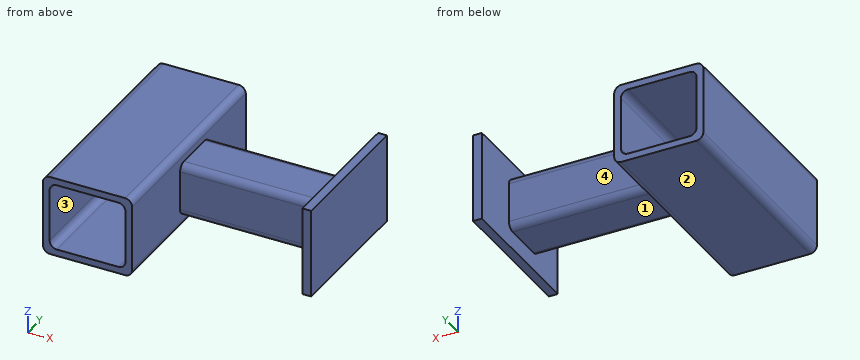
from build123d import *

# Parameters (mm, degrees)
F1_DEPTH = 152.4
F3_DEPTH = 101.6
F5_W     = 101.6
F5_H     = 63.5
F6_DEPTH = 6.35


with BuildPart() as f1:
    # F0 (on Front) → F1 (new body)
    with BuildSketch(Plane.XZ):
        with BuildLine():
            Line((-26.67, -28.575), (26.67, -28.575))
            ThreePointArc((26.67, -28.575), (30.2621024484, -27.0871024484), (31.75, -23.495))
            Line((31.75, -23.495), (31.75, 23.495))
            ThreePointArc((31.75, 23.495), (30.2621024484, 27.0871024484), (26.67, 28.575))
            Line((26.67, 28.575), (-26.67, 28.575))
            ThreePointArc((-26.67, 28.575), (-30.2621024484, 27.0871024484), (-31.75, 23.495))
            Line((-31.75, 23.495), (-31.75, -23.495))
            ThreePointArc((-31.75, -23.495), (-30.2621024484, -27.0871024484), (-26.67, -28.575))
        make_face()
        with BuildLine():
            Line((-21.9075, 23.8125), (21.9075, 23.8125))
            ThreePointArc((21.9075, 23.8125), (25.4996024484, 22.3246024484), (26.9875, 18.7325))
            Line((26.9875, 18.7325), (26.9875, -18.7325))
            ThreePointArc((26.9875, -18.7325), (25.4996024484, -22.3246024484), (21.9075, -23.8125))
            Line((21.9075, -23.8125), (-21.9075, -23.8125))
            ThreePointArc((-21.9075, -23.8125), (-25.4996024484, -22.3246024484), (-26.9875, -18.7325))
            Line((-26.9875, -18.7325), (-26.9875, 18.7325))
            ThreePointArc((-26.9875, 18.7325), (-25.4996024484, 22.3246024484), (-21.9075, 23.8125))
        make_face(mode=Mode.SUBTRACT)
    extrude(amount=-F1_DEPTH)

    # F2 (on face) → F3 (join)
    with BuildSketch(Plane.YZ.offset(31.75)):
        with BuildLine():
            Line((69.4262681528, -19.05), (97.3662681528, -19.05))
            ThreePointArc((97.3662681528, -19.05), (100.9583706013, -17.5621024484), (102.4462681528, -13.97))
            Line((102.4462681528, -13.97), (102.4462681528, 13.97))
            ThreePointArc((102.4462681528, 13.97), (100.9583706013, 17.5621024484), (97.3662681528, 19.05))
            Line((97.3662681528, 19.05), (69.4262681528, 19.05))
            ThreePointArc((69.4262681528, 19.05), (65.8341657044, 17.5621024484), (64.3462681528, 13.97))
            Line((64.3462681528, 13.97), (64.3462681528, -13.97))
            ThreePointArc((64.3462681528, -13.97), (65.8341657044, -17.5621024484), (69.4262681528, -19.05))
        make_face()
        with BuildLine():
            ThreePointArc((69.9342681528, -16.002), (68.1382169286, -15.2580512242), (67.3942681528, -13.462))
            Line((67.3942681528, -13.462), (67.3942681528, 13.462))
            ThreePointArc((67.3942681528, 13.462), (68.1382169286, 15.2580512242), (69.9342681528, 16.002))
            Line((69.9342681528, 16.002), (96.8582681528, 16.002))
            ThreePointArc((96.8582681528, 16.002), (98.6543193771, 15.2580512242), (99.3982681528, 13.462))
            Line((99.3982681528, 13.462), (99.3982681528, -13.462))
            ThreePointArc((99.3982681528, -13.462), (98.6543193771, -15.2580512242), (96.8582681528, -16.002))
            Line((96.8582681528, -16.002), (69.9342681528, -16.002))
        make_face(mode=Mode.SUBTRACT)
    extrude(amount=F3_DEPTH)

    # F4 (on face) + F5 (on face) → F6 (join)
    with BuildSketch(Plane.YZ.offset(133.35)):
        with BuildLine():
            ThreePointArc((64.3462681528, -13.97), (65.8341657044, -17.5621024484), (69.4262681528, -19.05))
            Line((69.4262681528, -19.05), (97.3662681528, -19.05))
            ThreePointArc((97.3662681528, -19.05), (100.9583706013, -17.5621024484), (102.4462681528, -13.97))
            Line((102.4462681528, -13.97), (102.4462681528, 13.97))
            ThreePointArc((102.4462681528, 13.97), (100.9583706013, 17.5621024484), (97.3662681528, 19.05))
            Line((97.3662681528, 19.05), (69.4262681528, 19.05))
            ThreePointArc((69.4262681528, 19.05), (65.8341657044, 17.5621024484), (64.3462681528, 13.97))
            Line((64.3462681528, 13.97), (64.3462681528, -13.97))
        make_face()
        with BuildLine():
            ThreePointArc((99.3982681528, -13.462), (98.6543193771, -15.2580512242), (96.8582681528, -16.002))
            Line((96.8582681528, -16.002), (69.9342681528, -16.002))
            ThreePointArc((69.9342681528, -16.002), (68.1382169286, -15.2580512242), (67.3942681528, -13.462))
            Line((67.3942681528, -13.462), (67.3942681528, 13.462))
            ThreePointArc((67.3942681528, 13.462), (68.1382169286, 15.2580512242), (69.9342681528, 16.002))
            Line((69.9342681528, 16.002), (96.8582681528, 16.002))
            ThreePointArc((96.8582681528, 16.002), (98.6543193771, 15.2580512242), (99.3982681528, 13.462))
            Line((99.3982681528, 13.462), (99.3982681528, -13.462))
        make_face(mode=Mode.SUBTRACT)
        with BuildLine():
            Line((69.9342681528, -16.002), (96.8582681528, -16.002))
            ThreePointArc((96.8582681528, -16.002), (98.6543193771, -15.2580512242), (99.3982681528, -13.462))
            Line((99.3982681528, -13.462), (99.3982681528, 13.462))
            ThreePointArc((99.3982681528, 13.462), (98.6543193771, 15.2580512242), (96.8582681528, 16.002))
            Line((96.8582681528, 16.002), (69.9342681528, 16.002))
            ThreePointArc((69.9342681528, 16.002), (68.1382169286, 15.2580512242), (67.3942681528, 13.462))
            Line((67.3942681528, 13.462), (67.3942681528, -13.462))
            ThreePointArc((67.3942681528, -13.462), (68.1382169286, -15.2580512242), (69.9342681528, -16.002))
        make_face()
    with BuildSketch(Plane.YZ.offset(133.35)):
        with Locations((87.8347480977, 0)):
            Rectangle(F5_W, F5_H)
        with BuildLine():
            ThreePointArc((102.4462681528, -13.97), (100.9583706013, -17.5621024484), (97.3662681528, -19.05))
            Line((97.3662681528, -19.05), (69.4262681528, -19.05))
            ThreePointArc((69.4262681528, -19.05), (65.8341657044, -17.5621024484), (64.3462681528, -13.97))
            Line((64.3462681528, -13.97), (64.3462681528, 13.97))
            ThreePointArc((64.3462681528, 13.97), (65.8341657044, 17.5621024484), (69.4262681528, 19.05))
            Line((69.4262681528, 19.05), (97.3662681528, 19.05))
            ThreePointArc((97.3662681528, 19.05), (100.9583706013, 17.5621024484), (102.4462681528, 13.97))
            Line((102.4462681528, 13.97), (102.4462681528, -13.97))
        make_face(mode=Mode.SUBTRACT)
    extrude(amount=F6_DEPTH)


solid = f1.part
CAD build for the part. Positions are in the model's coordinates, mm. Face numbers are marked on the shaded views. A direction names the side the tool comes from. Give positions to 0.01 mm unless a question says otherwise; leave off trailing zeros. Loops run counter-clockwise (first coordinate to the right, second up) from the corner with the lowest first, then second, coordinate; pieces in that order, holes last. Notation, with made-up numbers: M 54,23 L 65,23 A37 ccw 65,60 Z; hole C -24.5,85 d6. An arc over 180 degrees is marked long. One line per question, with ' | ' between items. Start each with the question number.
1. Saw through at B-B on x = -20. Give the cut face in (y, z) (1 decimal), plus the area to 3 significant figures.
2. Flat gauge pins, fed straight in: pin 1 (2 mm diameter, centred on x = 121, y = 85.5, fed in from +Z); pin 2 (5 mm diameter, centred on x = 28, z = -7, fed in from -Y); pin 3 (8 mm diameter, centred on x = 86.5, y = 86, fed in from -Z); pin 4 (13 mm diameter, centred on x = -9, y = 95.5, fed in from +Z) (3 decimals). Where does each tip first touch, or does it go through?
3. 3-axis set-ups, long thin cutter, end or side, ignore diameter. For the marked faces 1, 2, 3 and 4: which of +Z, -Z, +X, -X, +Y, -Y reach the whole face in a straight line?
4. Probe L1, parallel to X at y = 71, z = 9.5; L2, parallel to Z at x = 16.5, y = 49 (1 decimal); L3, parallel to Y at x = 88, z = 11. List the from-to ranges inside material, lowest first. Write a range as from..to.
5. Saw through at A-A on y = 41. State how many separate pieces and enclosed holes the cut face has, plus the area to 3 significant figures.
6. Saw through at C-C on x = 39.5. Give the cut face in (y, z), plus the area to 3 significant figures.
Result sheet:
1) outline: M 0,-28.6 L 152.4,-28.6 L 152.4,-23.8 L 0,-23.8 Z; M 0,23.8 L 152.4,23.8 L 152.4,28.6 L 0,28.6 Z | area: 1,450 mm^2
2) pin 1: stops at z = 19.05 | pin 2: stops at y = 0 | pin 3: stops at z = -19.05 | pin 4: stops at z = 28.575
3) face 1: -Z, +Y, -Y | face 2: -Z, -X, +Y, -Y | face 3: +Y, -Y | face 4: +Z, -Z, +Y
4) L1: x = -31.75..-26.99, 26.99..31.75, 133.35..139.7 | L2: z = -28.6..-23.8, 23.8..28.6 | L3: y = 64.35..67.39, 99.4..102.45
5) separate pieces: 2 | enclosed holes: 1 | area: 1,460 mm^2
6) outline: M 64.35,-13.97 A5.08 ccw 69.43,-19.05 L 97.37,-19.05 A5.08 ccw 102.45,-13.97 L 102.45,13.97 A5.08 ccw 97.37,19.05 L 69.43,19.05 A5.08 ccw 64.35,13.97 Z; hole M 67.39,-13.46 A2.54 ccw 69.93,-16 L 96.86,-16 A2.54 ccw 99.4,-13.46 L 99.4,13.46 A2.54 ccw 96.86,16 L 69.93,16 A2.54 ccw 67.39,13.46 Z | area: 411 mm^2
